```python
from build123d import *

# Parameters (mm, degrees)
BOSS_EXTRUDE1_DEPTH = 1.524
SKETCH4_R           = 1.143
CUT_EXTRUDE6_DEPTH  = 28.702


with BuildPart() as part:
    # Sketch1 → Boss-Extrude1 (new body)
    with BuildSketch(Plane.XY):
        with BuildLine():
            Line((6.7691, -2.7559), (-6.7691, -2.7559))
            ThreePointArc((-6.7691, -2.7559), (-9.525, 0), (-6.7691, 2.7559))
            Line((-6.7691, 2.7559), (6.7691, 2.7559))
            ThreePointArc((6.7691, 2.7559), (9.525, 0), (6.7691, -2.7559))
        make_face()
    extrude(amount=BOSS_EXTRUDE1_DEPTH)

    # Sketch2 → Revolve2 (revolve)
    with BuildSketch(Plane(origin=(0, 0, 0), x_dir=(1, 0, 0), z_dir=(0, 1, 0)), mode=Mode.PRIVATE) as revolve2_sk:
        with BuildLine():
            Line((0, 0), (6.096, 0))
            Line((6.096, 0), (6.096, -4.318))
            ThreePointArc((6.096, -4.318), (4.384917816, -8.448917816), (0.254, -10.16))
            Line((0.254, -10.16), (0, -10.16))
            Line((0, -10.16), (0, 0))
        make_face()
    revolve(revolve2_sk.sketch.rotate(Axis((0, 0, 0), (0, 0, 1)), 180), axis=Axis((0, 0, 0), (0, 0, 1)))

    # Sketch4 → Cut-Extrude6 (cut)
    with BuildSketch(Plane.XY):
        with Locations((-6.7691, 0)):
            Circle(SKETCH4_R)
        with Locations(Location((6.7691, 0, 0), (0, 0, 130.093582501))):
            Circle(SKETCH4_R)
    extrude(amount=CUT_EXTRUDE6_DEPTH, mode=Mode.SUBTRACT)


solid = part.part
```
For this review, take the finished solid that the model builds, in its own axes (mm). A direction names the side the tool comes from. Round coordinates to 2 decimals unless told otherwise and drop trailing zeros. Write each loop counter-clockwise with the first axis right and the second up, starting at its lowest first coordinate (ties: lowest second). Pieces come first, ordered by that corner, then holes. Notation, with made-up numbers: (3.5, 33.25) -> (8.5, 33.25) arc R20 cw to (8.5, 47.25) -> close; hole circle Ø1 at (23.25, 5). An arc over 180 degrees is marked (long way). Use one line per item in the form item = value.
Q1. To check wall thickness, follow probe 1 along Y at (x, z) = (-0.75, 6.5); probe 2 along Z at (x, y) = (-8.5, 1.5); probe 3 along X at (y, z) = (0, 4.25). State the ranges of each line that lie inside material, in increasing order. Write a range as from..to.
Resolved:
probe_1 = -5.62..5.62
probe_2 = 0..1.52
probe_3 = -5.63..5.63
Q2. The part is to be moulded in two halves that separate along Y. For faces 1 (the cylindrical face through (-9.524, -0.061, 0.751)), 2 (the cylindrical face through (-5.7, -0.4, 1.8)), 3 (the flat face through (6, -2.756, 1)), 4 (the flat face through (6, 2.756, 1)), say which applies: released by +Y, released by -Y, zero draft, split by the parting line, or undercut.
Resolved:
face_1 = split by the parting line
face_2 = undercut
face_3 = released by -Y
face_4 = released by +Y
Q3. Consider section B-B (y = 0). State how many separate pieces and enclosed holes the cut face has, then the cut area to 3 significant figures.
Resolved:
separate_pieces = 3
enclosed_holes = 0
area = 109 mm²
Q4. Machinability: for faces 5 (the flat face through (-6, 2.756, 1)), 6 (the flat face through (-6, -2.756, 1)), 7 (the cylindrical face through (0.122, 6.095, 2.189)), 8 (the cylindrical face through (-0.122, -6.095, 2.189)), 9 (the flat face through (0, 0, 0)), which of the approach directions +Z, -Z, +X, -X, +Y, -Y give a long, thin tool a straight path to every point of the face, cutting with its end or side? Answer none if there is none.
Resolved:
face_5 = +Z, -Z, -X, +Y
face_6 = +Z, -Z, -X, -Y
face_7 = +Z, +Y
face_8 = +Z, -Y
face_9 = -Z, +X, -X, +Y, -Y
Q5. Clearance check with flat-ended pins moving along their axes: pin 1 Ø1.5 at (x, z) = (6.5, 1) entering from +Y; pin 2 Ø6 at (y, z) = (3, 5) entering from +X; pin 3 Ø1.8 at (x, y) = (-6.77, 0) entering from -Z; pin 4 Ø2.5 at (x, y) = (6.77, 0) entering from +Z. State where each tip first meets the part, or that it passes through.
Resolved:
pin_1 = 2.76
pin_2 = 6.03
pin_3 = through
pin_4 = 6.85
Q6. Consider section A-A (x = -7.25). State the section outline as (y, z) points.
Resolved:
outline = (-2.71, 0) -> (-1.04, 0) -> (-1.04, 1.52) -> (-2.71, 1.52) -> close; (1.04, 0) -> (2.71, 0) -> (2.71, 1.52) -> (1.04, 1.52) -> close
